The listing builds one solid part. Answer for the finished solid, in the listing's coordinates (mm). A direction names the side the tool comes from. Coordinates: 2 decimals unless noted, no trailing zeros. Order: outer loops, then holes, each group sorted by start corner. A loop starts at its lowest first (then second) coordinate and runs counter-clockwise, first axis right, second up.
```python
from build123d import *

# Parameters (mm, degrees)
BOX010_W               = 200
BOX010_H               = 100
BOX010_DEPTH           = 100
BOX008_W               = 20
BOX008_H               = 20
BOX008_DEPTH           = 20
BOX008_PLACEMENT_ANGLE = 30
BOX011_W               = 14
BOX011_H               = 14
BOX011_DEPTH           = 20
SKETCH039_R            = 5.5
POCKET007_DEPTH        = 20.001
BOX014_W               = 7.5
BOX014_H               = 60
BOX014_DEPTH           = 200
ARRAY002_X_COUNT       = 7
ARRAY002_X_PITCH       = 47
BOX006_W               = 37
BOX006_H               = 60
BOX006_DEPTH           = 200
ARRAY_X_COUNT          = 6
ARRAY_X_PITCH          = 47
BOX012_W               = 14
BOX012_H               = 14
BOX012_DEPTH           = 12
SKETCH032_R            = 5.5
POCKET009_DEPTH        = 12.001
BOX013_W               = 14
BOX013_H               = 14
BOX013_DEPTH           = 12
SKETCH034_R            = 5.5
POCKET008_DEPTH        = 12.001
BOX009_W               = 37
BOX009_H               = 60
BOX009_DEPTH           = 200
ARRAY001_X_COUNT       = 6
ARRAY001_X_PITCH       = 47
SKETCH035_W            = 3
SKETCH035_H            = 4
SKETCH036_R            = 1.2
POCKET006_DEPTH        = 3.001
SKETCH037_W            = 5
SKETCH037_H            = 3.1
PAD022_DEPTH           = 5


with BuildPart() as bigleft:
    # Box010 → Box010 (new body)
    with BuildSketch(Plane(origin=(0, -50, -50), x_dir=(1, 0, 0), z_dir=(0, 0, 1))):
        with Locations((100, 50)):
            Rectangle(BOX010_W, BOX010_H)
    extrude(amount=BOX010_DEPTH)


with BuildPart() as pillar_cut_cube_l:
    # Box008 → Box008 (new body)
    with BuildSketch(Plane.XY):
        with Locations((10, 10)):
            Rectangle(BOX008_W, BOX008_H)
    extrude(amount=BOX008_DEPTH)


with BuildPart() as pillar_cut_cube_l_1:
    # Box008 placement: moved
    add(pillar_cut_cube_l.part.moved(Location((-127.001, 5, 20.4905))).rotate(Axis((-127.001, 5, 20.4905), (0, 1, 0)), BOX008_PLACEMENT_ANGLE))


with BuildPart() as cut011:
    # Box011 → Box011 (new body)
    with BuildSketch(Plane(origin=(-125, 8.55, 0), x_dir=(1, 0, 0), z_dir=(0, 0, 1))):
        with Locations((7, 7)):
            Rectangle(BOX011_W, BOX011_H)
    extrude(amount=BOX011_DEPTH)

    # Sketch039 → Pocket007 (cut, through all)
    with BuildSketch(Plane(origin=(-125, 8.55, 20), x_dir=(1, 0, 0), z_dir=(0, 0, 1))):
        with Locations((7, 7)):
            Circle(SKETCH039_R)
    extrude(amount=-POCKET007_DEPTH, mode=Mode.SUBTRACT)

    # Cut011: cut pillar_cut_cube_l
    add(pillar_cut_cube_l_1.part, mode=Mode.SUBTRACT)


with BuildPart() as array002:
    # Box014 → Box014 (new body)
    with BuildSketch(Plane(origin=(-128.8, 18.55, -100), x_dir=(1, 0, 0), z_dir=(0, 0, 1))):
        with Locations((3.75, 30)):
            Rectangle(BOX014_W, BOX014_H)
    extrude(amount=BOX014_DEPTH)

    # Array002 X: Array002 ×7


with BuildPart() as array002_1:
    add(array002.part)
    with Locations(*[(i * ARRAY002_X_PITCH, 0, 0) for i in range(1, ARRAY002_X_COUNT)]):
        add(array002.part)


with BuildPart() as rail_cut_cube_array_b:
    # Box006 → Box006 (new body)
    with BuildSketch(Plane(origin=(-120, 18.55, -100), x_dir=(1, 0, 0), z_dir=(0, 0, 1))):
        with Locations((18.5, 30)):
            Rectangle(BOX006_W, BOX006_H)
    extrude(amount=BOX006_DEPTH)

    # Array X: rail_cut_cube_array_b ×6


with BuildPart() as rail_cut_cube_array_b_1:
    add(rail_cut_cube_array_b.part)
    with Locations(*[(i * ARRAY_X_PITCH, 0, 0) for i in range(1, ARRAY_X_COUNT)]):
        add(rail_cut_cube_array_b.part)


with BuildPart() as cut013:
    # Sweep002: sweep along a path in Sketch028
    with BuildLine(Plane.XZ) as sweep002_path:
        Line((164.641016, 24.27441), (144.641016, 24.27441))
        ThreePointArc((144.641016, 24.27441), (123.935493, 21.548477), (104.641016, 13.556443))
        Line((104.641016, 13.556443), (70, -6.443557))
        ThreePointArc((70, -6.443557), (0, -25.2), (-70, -6.443557))
        Line((-70, -6.443557), (-130.621778, 28.556443))
    # Sketch043 → Sweep002 (sweep)
    with BuildSketch(Plane.YZ.offset(164.641016)):
        Polygon((18.55, 17.58), (47.05, 23.28), (18.55, 23.28), align=None)
    sweep(path=sweep002_path.line)

    # Cut012: cut rail_cut_cube_array_b
    add(rail_cut_cube_array_b_1.part, mode=Mode.SUBTRACT)

    # Cut013: cut Array002
    add(array002_1.part, mode=Mode.SUBTRACT)


with BuildPart() as rail_cut_b:
    # Sweep: sweep along a path in Sketch028
    with BuildLine(Plane.XZ) as sweep_path:
        Line((164.641016, 24.27441), (144.641016, 24.27441))
        ThreePointArc((144.641016, 24.27441), (123.935493, 21.548477), (104.641016, 13.556443))
        Line((104.641016, 13.556443), (70, -6.443557))
        ThreePointArc((70, -6.443557), (0, -25.2), (-70, -6.443557))
        Line((-70, -6.443557), (-130.621778, 28.556443))
    # Sketch029 → Sweep (sweep)
    with BuildSketch(Plane.YZ):
        Polygon((-19.25, -25.2), (-19.25, -31.9), (-9.25, -31.9), (-9.25, -26.2), (19.25, -26.2), (19.25, -25.2), align=None)
    sweep(path=sweep_path.line)


with BuildPart() as rail_cut_b_1:
    # Sweep placement: moved
    add(rail_cut_b.part.moved(Location((0, 27.8, 0))))

    # Cut007: cut rail_cut_cube_array_b
    add(rail_cut_cube_array_b_1.part, mode=Mode.SUBTRACT)


with BuildPart() as pillar_hollow_r:
    # Box012 → Box012 (new body)
    with BuildSketch(Plane(origin=(143, 8.55, 7), x_dir=(1, 0, 0), z_dir=(0, 0, 1))):
        with Locations((7, 7)):
            Rectangle(BOX012_W, BOX012_H)
    extrude(amount=BOX012_DEPTH)

    # Sketch032 → Pocket009 (cut, through all)
    with BuildSketch(Plane(origin=(143, 8.55, 19), x_dir=(1, 0, 0), z_dir=(0, 0, 1))):
        with Locations((7, 7)):
            Circle(SKETCH032_R)
    extrude(amount=-POCKET009_DEPTH, mode=Mode.SUBTRACT)


with BuildPart() as pillar_hollow_m:
    # Box013 → Box013 (new body)
    with BuildSketch(Plane(origin=(18, 8.55, -40), x_dir=(1, 0, 0), z_dir=(0, 0, 1))):
        with Locations((7, 7)):
            Rectangle(BOX013_W, BOX013_H)
    extrude(amount=BOX013_DEPTH)

    # Sketch034 → Pocket008 (cut, through all)
    with BuildSketch(Plane(origin=(18, 8.55, -28), x_dir=(1, 0, 0), z_dir=(0, 0, 1))):
        with Locations((7, 7)):
            Circle(SKETCH034_R)
    extrude(amount=-POCKET008_DEPTH, mode=Mode.SUBTRACT)


with BuildPart() as mount_cube_array_b:
    # Box009 → Box009 (new body)
    with BuildSketch(Plane(origin=(-120, 18.55, -100), x_dir=(1, 0, 0), z_dir=(0, 0, 1))):
        with Locations((18.5, 30)):
            Rectangle(BOX009_W, BOX009_H)
    extrude(amount=BOX009_DEPTH)

    # Array001 X: mount_cube_array_b ×6


with BuildPart() as mount_cube_array_b_1:
    add(mount_cube_array_b.part)
    with Locations(*[(i * ARRAY001_X_PITCH, 0, 0) for i in range(1, ARRAY001_X_COUNT)]):
        add(mount_cube_array_b.part)


with BuildPart() as mount_cube_array_b_2:
    # Array001 placement: moved
    add(mount_cube_array_b_1.part.moved(Location((0, -30, 0))))


with BuildPart() as cut014:
    # Sweep001: sweep along a path in Sketch028
    with BuildLine(Plane.XZ) as sweep001_path:
        Line((-130.621778, 28.556443), (-70, -6.443557))
        ThreePointArc((-70, -6.443557), (0, -25.2), (70, -6.443557))
        Line((70, -6.443557), (104.641016, 13.556443))
        ThreePointArc((104.641016, 13.556443), (123.935493, 21.548477), (144.641016, 24.27441))
        Line((144.641016, 24.27441), (164.641016, 24.27441))
    # Sketch035 → Sweep001 (sweep)
    with BuildSketch(Plane.YZ):
        with Locations((-17.75, -33.9)):
            Rectangle(SKETCH035_W, SKETCH035_H)
    sweep(path=sweep001_path.line)


with BuildPart() as cut014_1:
    # Sweep001 placement: moved
    add(cut014.part.moved(Location((0, 27.8, 0))))

    # Sketch036 → Pocket006 (cut, through all)
    with BuildSketch(Plane.XZ.offset(-8.55)):
        with Locations((-127.361382, 16.612761)):
            Circle(SKETCH036_R)
        with Locations((-78.25576, -11.759304)):
            Circle(SKETCH036_R)
        with Locations((-31.170284, -30.615305)):
            Circle(SKETCH036_R)
        with Locations((15.982787, -32.973976)):
            Circle(SKETCH036_R)
        with Locations((62.801571, -19.921701)):
            Circle(SKETCH036_R)
        with Locations((109.81105, 6.487408)):
            Circle(SKETCH036_R)
        with Locations((158.314011, 15.583238)):
            Circle(SKETCH036_R)
    extrude(amount=-POCKET006_DEPTH, mode=Mode.SUBTRACT)

    # Cut010: cut mount_cube_array_b
    add(mount_cube_array_b_2.part, mode=Mode.SUBTRACT)

    # Fusion003: union Cut011, Cut013, rail_cut_b, pillar_hollow_r, pillar_hollow_m
    add(cut011.part)
    add(cut013.part)
    add(rail_cut_b_1.part)
    add(pillar_hollow_r.part)
    add(pillar_hollow_m.part)

    # Cut014: cut bigleft
    add(bigleft.part, mode=Mode.SUBTRACT)


with BuildPart() as clone_of_fusion004:
    # Sketch037 → Pad022 (new body)
    with BuildSketch(Plane.YZ):
        with Locations((13.55, -28.55)):
            Rectangle(SKETCH037_W, SKETCH037_H)
    extrude(amount=PAD022_DEPTH)

    # Fusion004: union Cut014
    add(cut014_1.part)


with BuildPart() as obj1:
    # Part__Mirroring: instance of Clone of Fusion004
    add(clone_of_fusion004.part.mirror(Plane(origin=(0, 0, 0), x_dir=(1, 0, 0), z_dir=(0, 1, 0))))


with BuildPart() as obj1_1:
    # Part__Mirroring placement: moved
    add(obj1.part.moved(Location((0, -5, 0))))


solid = obj1_1.part
```
1) A cutting plane is placed at B-B, the plane x = -97. Write down the section's boundary in (y, z).
2) A cutting plane is placed at A-A, the plane y = -33. Write down the section's boundary in (x, z).
3) For faces 1 (the flat face through (-121.2, -25.3, 0)), 2 (the flat face through (2, -19, -27)), 3 (the flat face through (-79, -16.55, -13)), 4 (the flat face through (-74.3, -31, -7)), 5 (the flat face through (-26, -34, -25)), determine the directions among +Z, -Z, +X, -X, +Y, -Y from which every point of the face is accessible in a straight line to the end or side of a thin tool.
4) Straight lines are drawn through the part: probe 1 along Y at (x, z) = (-49, -19); probe 2 along Z at (x, y) = (-127, -15); probe 3 along Y at (x, z) = (-118, 12.25). For each, find the intervals that lie inside material, in ascending order.
5) The mould has two halves that part along Z. Classify faces 6 (the cylindrical face through (-31.09, -15.07, -32.66)), 7 (the flat face through (-36, -15, -30)), 8 (the cylindrical face through (-32.12, -15.03, -31.35)): released by +Z, released by -Z, zero draft, split by the parting line, or undercut.
6) Each of these flat-tipped pins is pushed along its axis until it touches: P1, Ø3.5, axis at y = -39, z = -26.5, coming from the +X side; P2, Ø2.5, axis at y = -15.5, z = -8.5, coming from the -X side; P3, Ø7, axis at y = -37.5, z = -8, coming from the -X side; P4, Ø2, axis at x = -31.17, z = -30.62, coming from the +Y side. Where does it stop, or does it pass through?
Working result:
1. outline: (-23.55, 1.41) - (-13.55, 1.41) - (-13.55, 9.14) - (-23.55, 9.14) - close
2. outline: (-133.02, 24.4) - (-128.8, 21.96) - (-128.8, 26.35) - (-121.3, 22.02) - (-121.3, 17.63) - (-120, 16.88) - (-120, 22.42) - (-130.62, 28.56) - close; (-83, -4.49) - (-81.8, -5.18) - (-81.8, -0.79) - (-74.3, -5.12) - (-74.3, -9.51) - (-73, -10.26) - (-73, -4.71) - (-83, 1.06) - close; (-36, -25.46) arc R144.8 ccw to (-34.8, -25.76) - (-34.8, -21.84) arc R141 ccw to (-27.3, -23.53) - (-27.3, -27.41) arc R144.8 ccw to (-26, -27.65) - (-26, -22.76) arc R140 cw to (-36, -20.49) - close
3. face 1: -Z, -X, +Y, -Y
3. face 2: +Z, +X, +Y, -Y
3. face 3: -Z, -X, -Y
3. face 4: -Z, -Y
3. face 5: +Z, -Z, +X, -Y
4. probe 1: y = -23.55 to -13.55
4. probe 2: z = 14.11 to 15.47, 17.76 to 26.47
4. probe 3: y = -27.55 to -26.05, -15.05 to -13.55
5. face 6: released by -Z
5. face 7: zero draft
5. face 8: undercut
6. P1: stops at x = -26
6. P2: stops at x = -83
6. P3: stops at x = -75.37
6. P4: passes through
